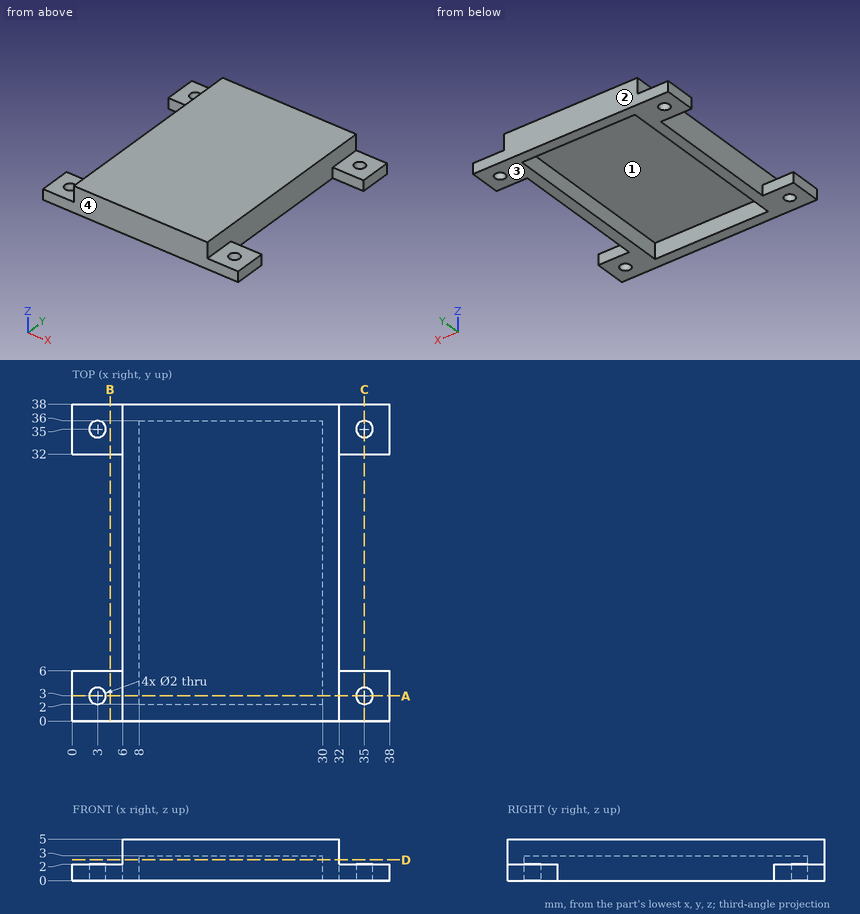
Check sheet for the drawn part. Datum: minimum x, y, z corner. Units: mm. Round coordinates to 2 decimals unless told otherwise and drop trailing zeros. Loops run counter-clockwise (first coordinate to the right, second up) from the corner with the lowest first, then second, coordinate; pieces in that order, holes last. Notation, with made-up numbers: (-26, 22.5) - (17, 22.5) arc R36 cw to (17, 60.5) - close; hole circle Ø9 at (82.25, 2.5). An arc over 180 degrees is marked (long way). Write each question's results on one line, items separated by ' | '. Start each with the question number.
Q1. Gauge pin test, flat ends, axial feed: P1, Ø1.5, axis at y = 17.5, z = 2, coming from the +X side; P2, Ø1.8, axis at x = 33.5, y = 34, coming from the +Z side; P3, Ø0.9, axis at y = 26, z = 1.5, coming from the -X side. Record the tip position at first contact, or that the pin passes through.
Q2. Thickness scan on line 1 (X direction, y = 35, z = 1.25); line 2 (Y direction, x = 3, z = 0.6); line 3 (Y direction, x = 23.5, z = 1.1). Record the ranges inside material, lowest first. Write a range as [from, to].
Q3. Cross-section at D-D on z = 2.5. Enter the section's corners in (x, y).
Q4. Cross-section at B-B on x = 4.5. Enter the section's corners in (y, z), and give its area (3 significant figures).
Q5. Cross-section at A-A on y = 3. Enter the section's corners in (x, z), and give its area (3 significant figures).
Q6. Cross-section at C-C on x = 35. Enter the section's corners in (y, z).
Q7. Release check for a two-part mould opening along Y. For the marked faces 1, 2, 3 and 4 record: +Y half, -Y half, draft (parallel to the pull), parting line (faces both ways), or undercut.
Answers below:
1) P1: stops at x = 32 | P2: stops at z = 2 | P3: stops at x = 6
2) line 1: x = [0, 2], [4, 8], [30, 34], [36, 38] | line 2: y = [0, 2], [4, 6], [32, 34], [36, 38] | line 3: y = [0, 2], [36, 38]
3) outline: (6, 0) - (32, 0) - (32, 38) - (6, 38) - close; hole (8, 2) - (30, 2) - (30, 36) - (8, 36) - close
4) outline: (0, 0) - (6, 0) - (6, 2) - (0, 2) - close; (32, 0) - (38, 0) - (38, 2) - (32, 2) - close | area: 24.0 mm²
5) outline: (0, 0) - (2, 0) - (2, 2) - (0, 2) - close; (4, 0) - (8, 0) - (8, 3) - (30, 3) - (30, 0) - (34, 0) - (34, 2) - (32, 2) - (32, 5) - (6, 5) - (6, 2) - (4, 2) - close; (36, 0) - (38, 0) - (38, 2) - (36, 2) - close | area: 80.0 mm²
6) outline: (0, 0) - (2, 0) - (2, 2) - (0, 2) - close; (4, 0) - (6, 0) - (6, 2) - (4, 2) - close; (32, 0) - (34, 0) - (34, 2) - (32, 2) - close; (36, 0) - (38, 0) - (38, 2) - (36, 2) - close
7) face 1: undercut | face 2: +Y half | face 3: draft | face 4: -Y half
